from build123d import *

# Parameters (mm, degrees)
EXTRUDE_1_DEPTH     = 2.9
EXTRUDE_2_DEPTH     = 80
CUT_EXTRUDE_1_DEPTH = 80
SKETCH_5_R          = 2.5
CUT_EXTRUDE_2_DEPTH = 80
EXTRUDE_START       = 1.5
EXTRUDE_3_DEPTH     = 1.5
SKETCH_8_R          = 2
CUT_EXTRUDE_3_DEPTH = 13
EXTRUDE_4_DEPTH     = 3.5
CUT_EXTRUDE_4_DEPTH = 50
CUT_EXTRUDE_5_DEPTH = 80


with BuildPart() as part:
    # 草图1 → 凸台-拉伸1 (new body)
    with BuildSketch(Plane(origin=(0, 0, 0), x_dir=(1, 0, 0), z_dir=(0, 1, 0))):
        with BuildLine():
            Line((-14.25, 8.5), (14.25, 8.5))
            ThreePointArc((14.25, 8.5), (19.906854249, 6.156854249), (22.25, 0.5))
            Line((22.25, 0.5), (22.25, -0.5))
            ThreePointArc((22.25, -0.5), (19.906854249, -6.156854249), (14.25, -8.5))
            Line((14.25, -8.5), (-14.25, -8.5))
            ThreePointArc((-14.25, -8.5), (-19.906854249, -6.156854249), (-22.25, -0.5))
            Line((-22.25, -0.5), (-22.25, 0.5))
            ThreePointArc((-22.25, 0.5), (-19.906854249, 6.156854249), (-14.25, 8.5))
        make_face()
    extrude(amount=EXTRUDE_1_DEPTH)

    # 草图3 → 凸台-拉伸2 (add)
    with BuildSketch(Plane(origin=(0, 2.9, 0), x_dir=(1, 0, 0), z_dir=(0, 1, 0))):
        with BuildLine():
            Line((-2.95, 6.95), (2.95, 6.95))
            ThreePointArc((2.95, 6.95), (6.485533906, 5.485533906), (7.95, 1.95))
            Line((7.95, 1.95), (7.95, -1.95))
            ThreePointArc((7.95, -1.95), (6.485533906, -5.485533906), (2.95, -6.95))
            Line((2.95, -6.95), (-2.95, -6.95))
            ThreePointArc((-2.95, -6.95), (-6.485533906, -5.485533906), (-7.95, -1.95))
            Line((-7.95, -1.95), (-7.95, 1.95))
            ThreePointArc((-7.95, 1.95), (-6.485533906, 5.485533906), (-2.95, 6.95))
        make_face()
    extrude(amount=EXTRUDE_2_DEPTH)

    # 草图4 → 切除-拉伸1 (cut)
    with BuildSketch(Plane(origin=(0, 82.9, 0), x_dir=(1, 0, 0), z_dir=(0, 1, 0))):
        with BuildLine():
            Line((5.95, -1.95), (5.95, 1.95))
            ThreePointArc((5.95, 1.95), (5.071320344, 4.071320344), (2.95, 4.95))
            Line((2.95, 4.95), (-2.95, 4.95))
            ThreePointArc((-2.95, 4.95), (-5.071320344, 4.071320344), (-5.95, 1.95))
            Line((-5.95, 1.95), (-5.95, -1.95))
            ThreePointArc((-5.95, -1.95), (-5.071320344, -4.071320344), (-2.95, -4.95))
            Line((-2.95, -4.95), (2.95, -4.95))
            ThreePointArc((2.95, -4.95), (5.071320344, -4.071320344), (5.95, -1.95))
        make_face()
    extrude(amount=-CUT_EXTRUDE_1_DEPTH, mode=Mode.SUBTRACT)

    # 草图5 → 切除-拉伸2 (cut)
    with BuildSketch(Plane(origin=(0, 2.9, 0), x_dir=(1, 0, 0), z_dir=(0, 1, 0))):
        with Locations(Location((-14.95, 0, 0), (0, 0, 270))):
            Circle(SKETCH_5_R)
        with Locations(Location((14.95, 0, 0), (0, 0, 270))):
            Circle(SKETCH_5_R)
    extrude(amount=-CUT_EXTRUDE_2_DEPTH, mode=Mode.SUBTRACT)

    # 草图7 → 凸台-拉伸3 (add)
    with BuildSketch(Plane(origin=(0, 0, 0), x_dir=(-1, 0, 0), z_dir=(0, -1, 0)).offset(EXTRUDE_START)):
        with BuildLine():
            Line((2.95, -6.95), (-2.95, -6.95))
            ThreePointArc((-2.95, -6.95), (-6.485533906, -5.485533906), (-7.95, -1.95))
            Line((-7.95, -1.95), (-7.95, 1.95))
            ThreePointArc((-7.95, 1.95), (-6.485533906, 5.485533906), (-2.95, 6.95))
            Line((-2.95, 6.95), (2.95, 6.95))
            ThreePointArc((2.95, 6.95), (6.485533906, 5.485533906), (7.95, 1.95))
            Line((7.95, 1.95), (7.95, -1.95))
            ThreePointArc((7.95, -1.95), (6.485533906, -5.485533906), (2.95, -6.95))
        make_face()
    extrude(amount=-EXTRUDE_3_DEPTH)

    # 草图8 → 切除-拉伸3 (cut)
    with BuildSketch(Plane.XY.offset(6.95)):
        with Locations((0, 75.720823604)):
            Circle(SKETCH_8_R)
        with Locations((0, 64.720823604)):
            Circle(SKETCH_8_R)
        with Locations((0, 53.720823604)):
            Circle(SKETCH_8_R)
        with Locations((0, 42.720823604)):
            Circle(SKETCH_8_R)
        with Locations((0, 31.720823604)):
            Circle(SKETCH_8_R)
        with Locations((0, 20.720823604)):
            Circle(SKETCH_8_R)
        with Locations((0, 9.720823604)):
            Circle(SKETCH_8_R)
    extrude(amount=-CUT_EXTRUDE_3_DEPTH, mode=Mode.SUBTRACT)

    # 草图9 → 凸台-拉伸4 (add, symmetric)
    with BuildSketch(Plane.ZY.offset(7.95)):
        Polygon((0, 17.081538124), (-6.397929019, 6), (6.397929019, 6), align=None)
    extrude_4 = extrude(amount=EXTRUDE_4_DEPTH, both=True)

    # 草图10 → 切除-拉伸4 (cut)
    with BuildSketch(Plane.XY.offset(6.95)):
        Polygon((-11.45, 6), (-7.95, 17.081538124), (-15.556844876, 23.601808742), align=None)
    cut_extrude_4 = extrude(amount=-CUT_EXTRUDE_4_DEPTH, mode=Mode.SUBTRACT)

    # 草图12 → 切除-拉伸5 (cut)
    with BuildSketch(Plane(origin=(0, 82.9, 0), x_dir=(1, 0, 0), z_dir=(0, 1, 0))):
        with BuildLine():
            Line((-2.95, -4.95), (2.95, -4.95))
            ThreePointArc((2.95, -4.95), (5.071320344, -4.071320344), (5.95, -1.95))
            Line((5.95, -1.95), (5.95, 1.95))
            ThreePointArc((5.95, 1.95), (5.071320344, 4.071320344), (2.95, 4.95))
            Line((2.95, 4.95), (-2.95, 4.95))
            ThreePointArc((-2.95, 4.95), (-5.071320344, 4.071320344), (-5.95, 1.95))
            Line((-5.95, 1.95), (-5.95, -1.95))
            ThreePointArc((-5.95, -1.95), (-5.071320344, -4.071320344), (-2.95, -4.95))
        make_face()
    cut_extrude_5 = extrude(amount=-CUT_EXTRUDE_5_DEPTH, mode=Mode.SUBTRACT)

    # 镜向2: 凸台-拉伸4 across plane
    add(extrude_4.mirror(Plane(origin=(0, 0, 0), x_dir=(0, 0, 1), z_dir=(1, 0, 0))))

    # 镜向3: 切除-拉伸4, 切除-拉伸5 across plane
    add(cut_extrude_4.mirror(Plane(origin=(0, 0, 0), x_dir=(0, 0, 1), z_dir=(1, 0, 0))), mode=Mode.SUBTRACT)
    add(cut_extrude_5.mirror(Plane(origin=(0, 0, 0), x_dir=(0, 0, 1), z_dir=(1, 0, 0))), mode=Mode.SUBTRACT)


solid = part.part
Check sheet for the modelled part. Datum: model origin and axes. Units: mm. A direction names the side the tool comes from. Round coordinates to 2 decimals unless told otherwise and drop trailing zeros. Loops run counter-clockwise (first coordinate to the right, second up) from the corner with the lowest first, then second, coordinate; pieces in that order, holes last. Notation, with made-up numbers: M 50.5,78 L 88.5,78 A21 cw 88.5,107 Z; hole C 17,-20.75 d9. An arc over 180 degrees is marked long. One line per item, written item: value.
(1) Thickness scan on line 1 (Z direction, x = 0.5, y = 79.5); line 2 (X direction, y = 39.5, z = -0.5). Record the ranges inside material, lowest first.
Computed values:
line 1: z = -6.95 to -4.95, 4.95 to 6.95
line 2: x = -7.95 to -5.95, 5.95 to 7.95
(2) Sectioned sample at A-A, the plane y = 47. Record the cut outline in (x, z).
Computed values:
outline: M -7.95,-1.95 A5 ccw -2.95,-6.95 L 2.95,-6.95 A5 ccw 7.95,-1.95 L 7.95,1.95 A5 ccw 2.95,6.95 L -2.95,6.95 A5 ccw -7.95,1.95 Z; hole M -5.95,-1.95 A3 ccw -2.95,-4.95 L 2.95,-4.95 A3 ccw 5.95,-1.95 L 5.95,1.95 A3 ccw 2.95,4.95 L -2.95,4.95 A3 ccw -5.95,1.95 Z
(3) Sectioned sample at D-D, the plane z = 4. Record the cut outline in (x, y), then the cut area to 3 significant figures.
Computed values:
outline: M -21.44,0 L -7.51,0 L -7.51,-1.5 L 7.51,-1.5 L 7.51,0 L 21.44,0 L 21.44,2.9 L 7.51,2.9 L 7.51,6 L 11.45,6 L 10.14,10.15 L 7.51,10.15 L 7.51,82.9 L 5.14,82.9 L 5.14,2.9 L -5.14,2.9 L -5.14,82.9 L -7.51,82.9 L -7.51,10.15 L -10.14,10.15 L -11.45,6 L -7.51,6 L -7.51,2.9 L -21.44,2.9 Z
area: 553 mm^2
(4) Access from +Z, -Z, +X, -X, +Y, -Y to the whole of each face (thin tool, end or side, straight path). Record for faces 4 (the face through (0, 82.9, 6)), 5 (the face through (-6.52, -0.76, 5.45)), 6 (the face through (-0.434, 73.768, -5.492)), 7 (the face through (-5.09, 43.46, 4.05)).
Computed values:
face 4: +Z, -Z, +X, -X, +Y
face 5: +Z, -X, -Y
face 6: +Z
face 7: +Y
(5) Sectioned sample at C-C, the plane x = 0. Count the separate pieces of the cut face and the enclosed holes in it, then the cut area to 3 significant figures.
Computed values:
separate pieces: 8
enclosed holes: 0
area: 303 mm^2
(6) Depth check by flat-ended pin: pin 1 Ø1 at (y, z) = (52.5, 0) entering from +X; pin 2 Ø5 at (x, z) = (-9, -1) entering from -Y; pin 3 Ø2.5 at (x, y) = (0, 64.72) entering from +Z; pin 4 Ø1 at (x, y) = (7.5, 35) entering from -Z. Enter the tip coordinate at first touch or a pass-through.
Computed values:
pin 1: stops at x = 7.95
pin 2: stops at y = -1.5
pin 3: stops at z = -6.05
pin 4: stops at z = -4.88
(7) Release check for a two-part mould opening along X. For faces 1 (the face through (6.45, -0.76, 5.52)), 2 (the face through (-19.969, 1.43, -6.094)), 3 (the face through (0, 32, -6.05)) record: +X half, -X half, draft (parallel to the pull), parting line (faces both ways), or undercut.
Computed values:
face 1: +X half
face 2: -X half
face 3: undercut
(8) Sectioned sample at B-B, the plane x = 10.5. Record the cut outline in (y, z), then the cut area to 3 significant figures.
Computed values:
outline: M 0,-8.5 L 2.9,-8.5 L 2.9,8.5 L 0,8.5 Z; M 6,-6.4 L 9.01,-4.66 L 9.01,4.66 L 6,6.4 Z
area: 82.6 mm^2
